Read the model definition and answer for the solid it produces. Units are mm, in the model's axes. A direction names the side the tool comes from. Coordinates: 2 decimals unless noted, no trailing zeros. Loops run counter-clockwise (first coordinate to the right, second up) from the corner with the lowest first, then second, coordinate; pieces in that order, holes last. Notation, with made-up numbers: (30, 83.25) -> (66, 83.25) arc R8 cw to (66, 95.25) -> close; hole circle Ø6 at (20.5, 87.25). An arc over 180 degrees is marked (long way). Answer as a JSON object with one key per item and string values. Group by question number.
1) Section C-C, the plane z = 0 is taken. Give the vertices of the cut face in (x, y).
2) Section D-D, the plane y = 59.5 is taken. Give the vertices of the cut face in (x, z).
3) Section B-B, the plane x = 0 is taken. Give the vertices of the cut face in (y, z).
4) Section A-A, the plane z = -8 is taken. Give the vertices of the cut face in (x, y), plus the area to 3 significant figures.
5) Determine the mould class of faces 1 (the face through (0, -75, 0)), 2 (the face through (-2.17, 62.32, -9.76)), 3 (the face through (-5, 50, -2)), 4 (the face through (-5, -50, -2)) for opening direction Y: released by +Y, released by -Y, zero draft, split by the parting line, or undercut.
6) Consider probe 1 along Y at (x, z) = (-3, 7.5); probe 2 along X at (y, z) = (-14.5, 0.5); probe 3 along Z at (x, y) = (0, -33.5). Determine where each line is inside the solid, lowest interval first. Write a range as [from, to].
7) Flat-ended cylindrical pins translate along their axes: P1, Ø4, axis at y = -22, z = 1, coming from the +X side; P2, Ø3, axis at x = -2, y = 0.5, coming from the +Z side; P3, Ø3, axis at x = 4, y = -4, coming from the +Z side. Find the tip coordinate at first contact, or state that the pin passes through.
8) Which of the six approach directions +Z, -Z, +X, -X, +Y, -Y give full straight-line access (tool end or side, diameter ignored) to faces 5 (the face through (-2.17, -62.32, -9.76)), 6 (the face through (-1.08, -0.7, -4.88))?
from build123d import *

# Parameters (mm, degrees)
F0_R          = 5
F1_DEPTH      = 50
F1_DEPTH_BACK = 50
F2_R          = 10
F3_DEPTH      = 25


# Not quite as in the source:
# - a pattern or mirror of a feature is missing from the dataset's text; its kind, count and spacing are read off the source's solid


with BuildPart() as f1:
    # F0 (on Front) → F1 (new body, two sides)
    with BuildSketch(Plane.XZ) as f1_sk:
        Circle(F0_R)
    extrude(amount=F1_DEPTH)
    extrude(f1_sk.sketch, amount=-F1_DEPTH_BACK)

    # F2 (on face) → F3 (join)
    with BuildSketch(Plane.XZ.offset(50)):
        Circle(F2_R)
    f3 = extrude(amount=F3_DEPTH)

    # F3_copies: F3 across plane
    add(f3.mirror(Plane.ZX))


solid = f1.part
Determined:
{
 "1": {"outline": "(-10, -75) -> (10, -75) -> (10, -50) -> (5, -50) -> (5, 50) -> (10, 50) -> (10, 75) -> (-10, 75) -> (-10, 50) -> (-5, 50) -> (-5, -50) -> (-10, -50) -> close"},
 "2": {"outline": "circle Ø20 at (0, 0)"},
 "3": {"outline": "(-75, -10) -> (-50, -10) -> (-50, -5) -> (50, -5) -> (50, -10) -> (75, -10) -> (75, 10) -> (50, 10) -> (50, 5) -> (-50, 5) -> (-50, 10) -> (-75, 10) -> close"},
 "4": {"outline": "(-6, -75) -> (6, -75) -> (6, -50) -> (-6, -50) -> close; (-6, 50) -> (6, 50) -> (6, 75) -> (-6, 75) -> close", "area": "600 mm²"},
 "5": {"face 1": "released by -Y", "face 2": "zero draft", "face 3": "undercut", "face 4": "undercut"},
 "6": {"probe 1": "[-75, -50], [50, 75]", "probe 2": "[-4.97, 4.97]", "probe 3": "[-5, 5]"},
 "7": {"P1": "x = 5", "P2": "z = 4.97", "P3": "z = 4.33"},
 "8": {"face 5": "+Y, -Y", "face 6": "none"}
}
